Autodesk Inventor part; units mm, degrees
ref_plane "YZ Plane" through (0, 0, 0) normal (1, 0, 0) x (0, 1, 0)
ref_plane "XZ Plane" through (0, 0, 0) normal (0, 1, 0) x (-1, 0, 0)
ref_plane "XY Plane" through (0, 0, 0) normal (0, 0, 1) x (1, 0, 0)
sketch "Esquisse1" plane through (0, 0, 0) normal (0, 1, 0) x (-1, 0, 0)
  line L0 (0, 0) -> (-18, 0)
  line L1 (-18, 0) -> (-18, -50)
  line L2 (-18, -50) -> (0, -50)
  line L3 (0, -50) -> (0, 0)
  dimension "d0" = 50
  dimension "d1" = 18
extrude "Extrusion1" add sketch "Esquisse1" along normal blind 13.6
sketch "Esquisse2" plane through (0, 0, 0) normal (0, -1, 0) x (1, 0, 0)
  line L0 (13.05, -10.6) -> (4.95, -10.6)
  line L1 (4.95, -10.6) -> (4.95, -27.6)
  line L2 (4.95, -39.4) -> (13.05, -39.4)
  line L3 (13.05, -39.4) -> (13.05, -31.4)
  line L4 (18, 0) -> (18, -50)
  line L5 (18, -25) -> (0, -25) construction
  line L6 (0, -50) -> (0, 0)
  line L7 (0, 0) -> (18, 0)
  line L8 (9, 0) -> (9, -50) construction
  line L9 (18, -50) -> (0, -50)
  line L10 (13.05, -31.4) -> (4.95, -31.4)
  line L11 (4.95, -27.6) -> (13.05, -27.6)
  line L12 (13.05, -31.4) -> (13.05, -27.6) construction
  line L13 (13.05, -27.6) -> (13.05, -10.6)
  line L14 (4.95, -27.6) -> (4.95, -31.4) construction
  line L15 (4.95, -31.4) -> (4.95, -39.4)
  point P0 (13.05, -25)
  point P1 (9, -10.6)
  dimension "d4" = 28.8
  dimension "d5" = 8.1
  dimension "d36" = 8
  dimension "d37" = 17
extrude "Extrusion2" cut sketch "Esquisse2" against normal blind 13.6 contours L13 L11 L1 L0 | L15 L10 L3 L2
sketch "Esquisse3" plane through (0, 0, 0) normal (0, -1, 0) x (1, 0, 0)
  circle A0 centre (9, -43.3) radius 1.75
  line L0 (4.95, -10.6) -> (13.05, -10.6)
  line L1 (0, -50) -> (0, 0)
  line L2 (18, -50) -> (0, -50)
  line L3 (9, -50) -> (9, 0)
  line L4 (0, 0) -> (18, 0)
  circle A1 centre (9, -6.7) radius 1.75
  line L5 (13.05, -39.4) -> (4.95, -39.4)
  dimension "d8" = 32.7
  dimension "d10" = 3.5
  dimension "d11" = 3.5
  dimension "d12" = 32.7
extrude "Extrusion3" cut sketch "Esquisse3" against normal blind 13.6 contours A0 L3 | L3 A0 | A1 L3 | L3 A1
sketch "Esquisse4" plane through (0, 0, 0) normal (0, -1, 0) x (1, 0, 0)
  line L0 (13.55, -10) -> (13.55, -40)
  line L1 (13.55, -40) -> (4.45, -40)
  line L2 (4.45, -40) -> (4.45, -30.5)
  line L3 (4.45, -30.5) -> (0, -30.5)
  line L4 (0, -30.5) -> (0, -19.5)
  line L5 (0, -50) -> (0, 0)
  line L6 (0, -19.5) -> (4.45, -19.5)
  line L7 (4.45, -19.5) -> (4.45, -10)
  line L8 (4.45, -10) -> (13.55, -10)
  line L9 (18, 0) -> (18, -50)
  line L10 (18, -25) -> (0, -25) construction
  line L11 (0, 0) -> (18, 0)
  line L12 (9, 0) -> (9, -50) construction
  line L13 (0, -50) -> (0, 0)
  point P0 (13.55, -25)
  point P1 (9, -10)
  dimension "d15" = 30
  dimension "d16" = 9.1
  dimension "d17" = 11
extrude "Extrusion4" cut sketch "Esquisse4" against normal blind 11.6
sketch "Esquisse5" plane through (0, 0, 0) normal (0, -1, 0) x (1, 0, 0)
  line L0 (16, -10) -> (16, -40)
  line L1 (16, -40) -> (13.25, -40)
  line L2 (13.25, -40) -> (13.25, -43)
  line L3 (13.25, -43) -> (4.75, -43)
  line L4 (4.75, -43) -> (4.75, -40)
  line L5 (4.75, -40) -> (2, -40)
  line L6 (2, -40) -> (2, -10)
  line L7 (2, -10) -> (4.75, -10)
  line L8 (4.75, -10) -> (4.75, -7)
  line L9 (4.75, -7) -> (13.25, -7)
  line L10 (13.25, -7) -> (13.25, -10)
  line L11 (16, -10) -> (13.25, -10)
  line L12 (0, 0) -> (18, 0)
  line L13 (9, 0) -> (9, -50)
  line L14 (18, -50) -> (0, -50)
  line L15 (0, -30.5) -> (0, -19.5)
  line L16 (0, -25) -> (9, -25)
  line L17 (4.45, -10) -> (13.55, -10)
  point P0 (2, -25)
  point P1 (9, -7)
  dimension "d20" = 14
  dimension "d21" = 36
  dimension "d22" = 8.5
extrude "Extrusion5" cut sketch "Esquisse5" against normal blind 7
sketch "Esquisse6" plane through (0, 0, 0) normal (0, -1, 0) x (1, 0, 0)
  circle A0 centre (9, -6.7) radius 4.25
  arc A1 (10.7241, -7) -> (7.2759, -7) centre (9, -6.7) ccw
  circle A2 centre (9, -43.3) radius 4.25
  arc A3 (10.7241, -43) -> (7.2759, -43) centre (9, -43.3) ccw
  point P0 (0, 0)
  dimension "d25" = 8.5
  dimension "d26" = 8.5
extrude "Extrusion6" cut sketch "Esquisse6" against normal blind 1.5
chamfer "Chanfrein1" distance 1.5 angle 45 1 edges at (7.25, 13.6, -6.7)
chamfer "Chanfrein2" distance 1.5 angle 45 1 edges at (7.25, 13.6, -43.3)
equation "\"d11\" = d10"
equation "\"d12\" = d8"
properties part number "sharp1"
Here's how the part is built. I have some questions about the finished solid (model axes, mm). A direction names the side the tool comes from. Coordinates: 2 decimals unless noted, no trailing zeros. Order: outer loops, then holes, each group sorted by start corner. A loop starts at its lowest first (then second) coordinate and runs counter-clockwise, first axis right, second up.
Item 1: If we mould it in two halves opening along Z, with no side actions, what happens to faces 3 (the face through (9, 7, -50)), 4 (the face through (1.7, 7, -19.5))? For each: +Z half, -Z half, draft (parallel to the pull), parting line (faces both ways), or undercut.
Result sheet:
face 3: -Z half
face 4: undercut
Item 2: For P1, Ø2.5, axis at x = 10, z = -8.5, coming from the -Y side; P2, Ø4, axis at x = 8.5, z = -35, coming from the -Y side; P3, Ø5.5, axis at x = 9, z = -6.7, coming from the -Y side, each with a flat end and sliding along its axis, tell me the tip position at first contact or that it passes through.
Result sheet:
P1: stops at y = 7
P2: passes through
P3: stops at y = 1.5
Item 3: I need wall thicknesses on line 1 (Z direction, x = 9, y = 7.25); line 2 (X direction, y = 10, z = -6.7); line 3 (Z direction, x = 2, y = 10.75). Which ranges of each line are inside material? Lowest first, please.
Result sheet:
line 1: z = -50 to -45.05, -41.55 to -40, -10 to -8.45, -4.95 to 0
line 2: x = 0 to 7.25, 10.75 to 18
line 3: z = -50 to -30.5, -19.5 to 0
Item 4: For faces 1 (the face through (9, 13, -31.4)), 2 (the face through (9.1, 0.74, -2.45)), which set-ups out of +Z, -Z, +X, -X, +Y, -Y let a thin tool reach every point of the face, with its end or its side?
Result sheet:
face 1: +Y, -Y
face 2: -Y
Item 5: If we section it at D-D on x = 3.5: List the corners of the cut face in (y, z) for me, plus the area to 3 significant figures.
Result sheet:
outline: (0, -50) - (13.6, -50) - (13.6, 0) - (0, 0) - (0, -10) - (7, -10) - (7, -19.5) - (11.6, -19.5) - (11.6, -30.5) - (7, -30.5) - (7, -40) - (0, -40) - close
area: 419 mm2
Item 6: If we section it at A-A on z = -21: List the corners of the cut face in (x, y) for me, plus the area to 3 significant figures.
Result sheet:
outline: (0, 11.6) - (4.95, 11.6) - (4.95, 13.6) - (0, 13.6) - close; (13.05, 11.6) - (13.55, 11.6) - (13.55, 7) - (16, 7) - (16, 0) - (18, 0) - (18, 13.6) - (13.05, 13.6) - close
area: 54.3 mm2
Item 7: If we section it at B-B on x = 9: State how many separate pieces and enclosed holes the cut face has, plus the area to 3 significant figures.
Result sheet:
separate pieces: 5
enclosed holes: 0
area: 153 mm2
Item 8: If we section it at C-C on y = 5.25: List the corners of the cut face in (x, z) for me, plus the area to 3 significant figures.
Result sheet:
outline: (0, -50) - (18, -50) - (18, 0) - (0, 0) - (0, -19.5) - (2, -19.5) - (2, -10) - (4.75, -10) - (4.75, -7) - (7.28, -7) arc R1.75 cw (long way) to (10.72, -7) - (13.25, -7) - (13.25, -10) - (16, -10) - (16, -40) - (13.25, -40) - (13.25, -43) - (10.72, -43) arc R1.75 cw (long way) to (7.28, -43) - (4.75, -43) - (4.75, -40) - (2, -40) - (2, -30.5) - (0, -30.5) - close
area: 395 mm2
